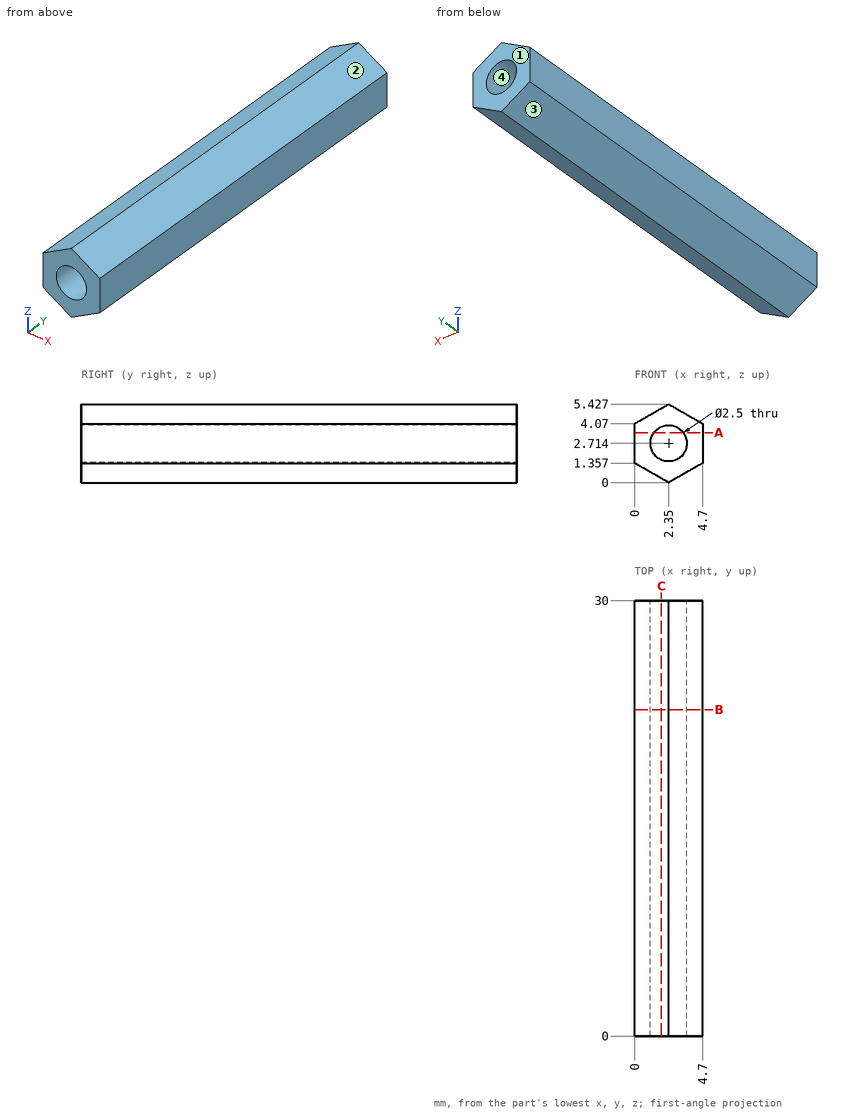
Part print with two shaded views. Sizes in mm from the minimum x, y, z corner. Coordinates: 2 decimals unless noted, no trailing zeros. Write each loop counter-clockwise with the first axis right and the second up, starting at its lowest first coordinate (ties: lowest second). Pieces come first, ordered by that corner, then holes. Notation, with made-up numbers: (-17, 84) - (-9, 84) arc R27 cw to (-9, 109) - close; hole circle Ø4 at (50.5, 78). An arc over 180 degrees is marked (long way). One line per item, written item: value. Start each with the question number.
1. Flat gauge pins, fed straight in: pin 1 (1.5 mm diameter, centred on x = 4, y = 26.5, fed in from -Z); pin 2 (2 mm diameter, centred on x = 4, y = 21, fed in from -Z) (1 decimal). Where does each tip first touch, or does it go through?
2. Slice it at A-A (z = 3.45). Write the cut outline in (x, y).
3. Slice it at B-B (y = 22.5). Write the cut outline in (x, z).
4. Slice it at C-C (x = 1.85). Write the cut outline in (y, z).
5. Mould opens along Z. For the marked faces 1, 2, 3 and 4 say: released by +Z, released by -Z, zero draft, split by the parting line, or undercut.
6. Probe line 1 (X direction, y = 26.25, z = 2.2); line 2 (X direction, y = 15.25, z = 2.1); line 3 (Z direction, x = 1.6, y = 7) (1 decimal). List the from-to ranges inside material, lowest first. Write a range as from..to.
Answers below:
1. pin 1: stops at z = 0.52
1. pin 2: stops at z = 0.4
2. outline: (0, 0) - (1.34, 0) - (1.34, 30) - (0, 30) - close; (3.36, 0) - (4.7, 0) - (4.7, 30) - (3.36, 30) - close
3. outline: (0, 1.36) - (2.35, 0) - (4.7, 1.36) - (4.7, 4.07) - (2.35, 5.43) - (0, 4.07) - close; hole circle Ø2.5 at (2.35, 2.71)
4. outline: (0, 0.29) - (30, 0.29) - (30, 1.57) - (0, 1.57) - close; (0, 3.86) - (30, 3.86) - (30, 5.14) - (0, 5.14) - close
5. face 1: zero draft
5. face 2: released by +Z
5. face 3: released by -Z
5. face 4: undercut
6. line 1: x = 0..1.21, 3.49..4.7
6. line 2: x = 0..1.26, 3.44..4.7
6. line 3: z = 0.4..1.7, 3.7..5
